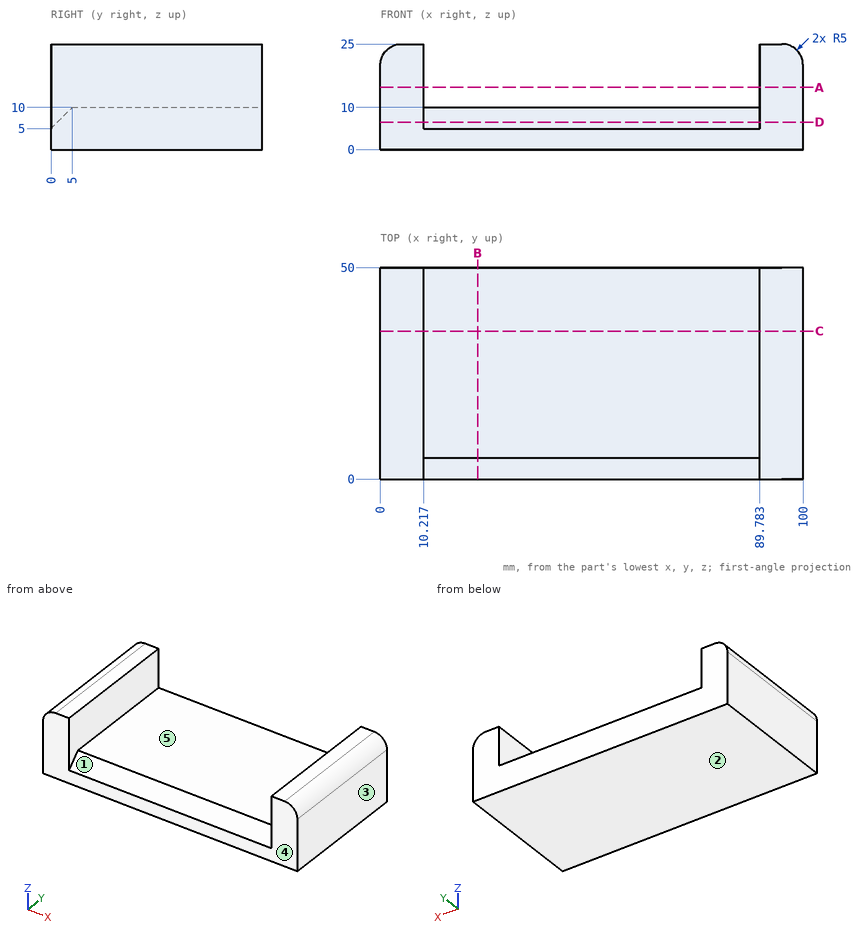
Design review of the part shown in the three views and the two pictorial views. Dimensions are in mm from the part's minimum x, y and z. A direction names the side the tool comes from. Round coordinates to 2 decimals unless told otherwise and drop trailing zeros. Loops run counter-clockwise (first coordinate to the right, second up) from the corner with the lowest first, then second, coordinate; pieces in that order, holes last. Notation, with made-up numbers: (-23.75, 61.25) - (-18.75, 61.25) arc R17 ccw to (-18.75, 85.25) - close; hole circle Ø5 at (-33.75, -37.5). An arc over 180 degrees is marked (long way). One line per item, written item: value. Start each with the question number.
Item 1: Clearance check with flat-ended pins moving along their axes: pin 1 Ø1.5 at (x, y) = (21, 15.5) entering from -Z; pin 2 Ø3 at (x, y) = (73, 31.5) entering from +Z; pin 3 Ø6 at (x, z) = (72.5, 15) entering from -Y. State where each tip first meets the part, or that it passes through.
Item 2: Take a section at A-A (z = 14.75). Give the boundary of the cut face in (x, y).
Item 3: Take a section at B-B (x = 23). Give the boundary of the cut face in (y, z).
Item 4: The part is to be moulded in two halves that separate along X. For the marked faces 3, 4 and 5, say which applies: +X half, -X half, draft (parallel to the pull), parting line (faces both ways), or undercut.
Item 5: For L1, parallel to X at y = 15.5, z = 16.5; L2, parallel to Z at x = 85, y = 29; L3, parallel to X at y = 45, z = 23.25 (1 decimal), list the stretches that pass through material, from the lowest coordinate up.
Item 6: For the marked faces 1 and 2, list the 3-axis set-ups (+Z, -Z, +X, -X, +Y, -Y) from which the entire face can be reached by the end or side of a thin tool; tool diameter is ignored.
Item 7: Take a section at D-D (z = 6.5). Give the boundary of the cut face in (x, y), plus the area to 3 significant figures.
Item 8: Take a section at C-C (y = 35). Give the boundary of the cut face in (x, z).
Answer below:
1. pin 1: stops at z = 0
1. pin 2: stops at z = 10
1. pin 3: passes through
2. outline: (0, 0) - (10.22, 0) - (10.22, 50) - (0, 50) - close; (89.78, 0) - (100, 0) - (100, 50) - (89.78, 50) - close
3. outline: (0, 0) - (50, 0) - (50, 10) - (5, 10) - (0, 5) - close
4. face 3: +X half
4. face 4: draft
4. face 5: undercut
5. L1: x = 0 to 10.22, 89.78 to 100
5. L2: z = 0 to 10
5. L3: x = 1.2 to 10.2, 89.8 to 98.8
6. face 1: +Z, -Y
6. face 2: -Z, +X, -X, +Y, -Y
7. outline: (0, 0) - (10.22, 0) - (10.22, 1.5) - (89.78, 1.5) - (89.78, 0) - (100, 0) - (100, 50) - (0, 50) - close
7. area: 4,880 mm2
8. outline: (0, 0) - (100, 0) - (100, 20) arc R5 ccw to (95, 25) - (89.78, 25) - (89.78, 10) - (10.22, 10) - (10.22, 25) - (5, 25) arc R5 ccw to (0, 20) - close
